from build123d import *

# Parameters (mm, degrees)
F1_DEPTH = 12.7
F2_DEPTH = 6.35
F3_DEPTH = 6.35
F4_DEPTH = 6.35


with BuildPart() as f1:
    # F0 (on Top) → F1 (new body)
    with BuildSketch(Plane.XY):
        Polygon((201.0800465941, 169.5929964036), (-256.1199534059, 169.5929964036), (-299.5649909763, -76.7960553225), (244.5250841646, -76.7960553225), align=None)
    extrude(amount=F1_DEPTH)

    # F2 (add): a face of the model
    f2_faces = [f1.faces().sort_by_distance(p)[0] for p in [
        (-27.5199534059, 42.8349405589, 12.7),
    ]]
    extrude(f2_faces, amount=-F2_DEPTH)

    # F3 (add): a face of the model
    f3_faces = [f1.faces().sort_by_distance(p)[0] for p in [
        (-27.5199534059, 42.8349405589, 12.7),
    ]]
    extrude(f3_faces, amount=-F3_DEPTH)

    # F4 (cut): a face of the model
    f4_faces = [f1.faces().sort_by_distance(p)[0] for p in [
        (-27.5199534059, 42.8349405589, 12.7),
    ]]
    extrude(f4_faces, amount=-F4_DEPTH, mode=Mode.SUBTRACT)


solid = f1.part
The listing builds one solid part. Answer for the finished solid, in the listing's coordinates (mm). Give positions to 0.01 mm unless a question says otherwise; leave off trailing zeros. Order: outer loops, then holes, each group sorted by start corner. A loop starts at its lowest first (then second) coordinate and runs counter-clockwise, first axis right, second up. Notation, with made-up numbers: (81.25, 50.5) - (137.25, 50.5) arc R20 cw to (137.25, 71.5) - close; hole circle Ø11 at (61, 4.5). An arc over 180 degrees is marked (long way). One line per item, written item: value. Start each with the question number.
1) A cutting plane is placed at B-B on y = 18. Give the vertices of the cut face in (x, z).
2) A cutting plane is placed at A-A on z = 2. Give the vertices of the cut face in (x, y) (3 decimals), then the cut area to 3 significant figures.
3) Find the intervals of material crossed by L1, parallel to X at y = -29, z = 1.5; L2, parallel to X at y = -27.5, z = 4.5, in increasing order.
4) Given pin 1 Ø2 at (x, y) = (-27, -2.5) entering from -Z; pin 2 Ø1 at (y, z) = (7, 3.5) entering from +X; pin 3 Ø1.5 at (y, z) = (110.5, 5) entering from -X; pin 4 Ø3 at (y, z) = (-10.5, 1) entering from +X, each flat-ended and moving along its own axis, determine where each tip first touches the part or whether it passes through.
Answer sheet:
1. outline: (-282.85, 0) - (227.81, 0) - (227.81, 6.35) - (-282.85, 6.35) - close
2. outline: (-299.565, -76.796) - (244.525, -76.796) - (201.08, 169.593) - (-256.12, 169.593) - close
2. area: 123,000 mm2
3. L1: x = -291.14 to 236.1
3. L2: x = -290.87 to 235.83
4. pin 1: stops at z = 0
4. pin 2: stops at x = 229.84
4. pin 3: stops at x = -266.67
4. pin 4: stops at x = 233.1
